from build123d import *

# Parameters (mm, degrees)
ESQUISSE1_W             = 45
ESQUISSE1_H             = 30
BOSS_EXTRU_1_DEPTH      = 25
ESQUISSE2_R             = 10
BOSS_EXTRU_2_DEPTH      = 30
ESQUISSE3_W             = 10
ESQUISSE3_H             = 4
BOSS_EXTRU_3_DEPTH      = 6
ESQUISSE4_R             = 1.5
ENL_V_MAT_EXTRU_1_DEPTH = 6
ESQUISSE6_W             = 10
ESQUISSE6_H             = 4
BOSS_EXTRU_4_DEPTH      = 6
ESQUISSE7_R             = 1.5
ENL_V_MAT_EXTRU_2_DEPTH = 6


with BuildPart() as part:
    # Esquisse1 → Boss.-Extru.1 (new body)
    with BuildSketch(Plane.XY):
        Rectangle(ESQUISSE1_W, ESQUISSE1_H)
    extrude(amount=BOSS_EXTRU_1_DEPTH)

    # Esquisse2 → Boss.-Extru.2 (add)
    with BuildSketch(Plane(origin=(0, 0, 0), x_dir=(-1, 0, 0), z_dir=(0, 0, -1))):
        with Locations((9.492124495, 0)):
            Circle(ESQUISSE2_R)
    extrude(amount=BOSS_EXTRU_2_DEPTH)

    # Esquisse3 → Boss.-Extru.3 (add)
    with BuildSketch(Plane.ZY.offset(22.5)):
        with Locations((20, -13)):
            Rectangle(ESQUISSE3_W, ESQUISSE3_H)
    extrude(amount=BOSS_EXTRU_3_DEPTH)

    # Esquisse4 → Enlèv. mat.-Extru.1 (cut)
    with BuildSketch(Plane(origin=(0, -11, 0), x_dir=(1, 0, 0), z_dir=(0, 1, 0))):
        with Locations(Location((-25.529560032, -20, 0), (0, 0, 270))):
            Circle(ESQUISSE4_R)
    extrude(amount=-ENL_V_MAT_EXTRU_1_DEPTH, mode=Mode.SUBTRACT)

    # Esquisse6 → Boss.-Extru.4 (add)
    with BuildSketch(Plane(origin=(0, 0, 0), x_dir=(-1, 0, 0), z_dir=(0, 0, -1))):
        with Locations((-17.5, -13)):
            Rectangle(ESQUISSE6_W, ESQUISSE6_H)
    extrude(amount=BOSS_EXTRU_4_DEPTH)

    # Esquisse7 → Enlèv. mat.-Extru.2 (cut)
    with BuildSketch(Plane(origin=(0, -11, 0), x_dir=(1, 0, 0), z_dir=(0, 1, 0))):
        with Locations(Location((17.789413963, 3, 0), (0, 0, 270))):
            Circle(ESQUISSE7_R)
    extrude(amount=-ENL_V_MAT_EXTRU_2_DEPTH, mode=Mode.SUBTRACT)


solid = part.part
Can you work these out from the model? Positions are in its coordinate system, mm. A direction names the side the tool comes from. Give positions to 0.01 mm unless a question says otherwise; leave off trailing zeros. Loops run counter-clockwise (first coordinate to the right, second up) from the corner with the lowest first, then second, coordinate; pieces in that order, holes last. Notation, with made-up numbers: (89, -32) - (128, -32) arc R15 cw to (128, -27) - close; hole circle Ø3 at (-17, -37.5). An arc over 180 degrees is marked (long way). One line per item, written item: value.
(1) If we section it at B-B, the plane y = 0: List the corners of the cut face in (x, z) for me, plus the area to 4 significant figures.
Verdict:
outline: (-22.5, 0) - (-19.49, 0) - (-19.49, -30) - (0.51, -30) - (0.51, 0) - (22.5, 0) - (22.5, 25) - (-22.5, 25) - close
area: 1,725 mm^2
(2) On a 3-axis mill with a long thin cutter (end or side, diameter ignored), from which of +Z, -Z, +X, -X, +Y, -Y can I reach the whole of each face in a straight line? I mean faces 1 (the face through (-27, -11, 19)), 2 (the face through (18, -13, -6)), 3 (the face through (0.5, 0.4, -14.8)), 4 (the face through (12.5, -13, -3)). Say none if no direction works.
Verdict:
face 1: +Z, -Z, -X, +Y
face 2: -Z, +X, -X, +Y, -Y
face 3: -Z
face 4: -Z, -X, +Y, -Y
(3) If we mould it in two halves opening along Z, with no side actions, what happens to faces 5 (the face through (16, -11, -2)), 6 (the face through (-25.5, -13, 18.5)), 7 (the face through (-3, 0, 25)), 8 (the face through (16.459, -12.972, -2.308))? For each: released by +Z, released by -Z, zero draft, split by the parting line, or undercut.
Verdict:
face 5: zero draft
face 6: undercut
face 7: released by +Z
face 8: undercut
(4) If we section it at A-A, the plane z = 20: List the corners of the cut face in (x, y) for me, plus the area to 3 significant figures.
Verdict:
outline: (-28.5, -15) - (-27.03, -15) - (-27.03, -11) - (-28.5, -11) - close; (-24.03, -15) - (22.5, -15) - (22.5, 15) - (-22.5, 15) - (-22.5, -11) - (-24.03, -11) - close
area: 1,360 mm^2
(5) I need wall thicknesses on line 1 along X through (y, z) = (-13.8, -3); line 2 along X through (y, z) = (-13.6, 20); line 3 along X through (y, z) = (8.75, 2). Which ranges of each line are inside material? Lowest first, please.
Verdict:
line 1: 12.5 to 16.29, 19.29 to 22.5
line 2: -28.5 to -27.03, -24.03 to 22.5
line 3: -22.5 to 22.5
(6) I'm going to push flat-ended pins straight in: pin 1 (4.5 mm diameter, centred on x = -24, y = -13, fed in from -Z); pin 2 (5 mm diameter, centred on x = 17.79, z = -3, fed in from +Y); pin 3 (1.2 mm diameter, centred on x = 19.5, y = -12, fed in from -Z); pin 4 (2.5 mm diameter, centred on x = -25.53, z = 20, fed in from +Y). Where does each tip first touch, or does it pass through?
Verdict:
pin 1: z = 0
pin 2: y = -11
pin 3: z = -6
pin 4: through
(7) If we section it at C-C, the plane z = -3: List the corners of the cut face in (x, y) for me, plus the area to 3 significant figures.
Verdict:
outline: circle Ø20 at (-9.49, 0); (12.5, -15) - (16.29, -15) - (16.29, -11) - (12.5, -11) - close; (19.29, -15) - (22.5, -15) - (22.5, -11) - (19.29, -11) - close
area: 342 mm^2
(8) If we section it at D-D, the plane x = -11: List the corners of the cut face in (y, z) for me.
Verdict:
outline: (-15, 0) - (-9.89, 0) - (-9.89, -30) - (9.89, -30) - (9.89, 0) - (15, 0) - (15, 25) - (-15, 25) - close
